from build123d import *

# Parameters (mm, degrees)
SKETCH_1_W                      = 90
SKETCH_1_H                      = 90
EXTRUDE_1_DEPTH                 = 15
SKETCH_2_W                      = 5
SKETCH_2_H                      = 82.5
CUT_EXTRUDE_1_DEPTH             = 102.734949747
CUT_EXTRUDE_2_REACH             = 67.383
SKETCH_3_W                      = 40
SKETCH_3_H                      = 90
FILLET_1_R                      = 10
CUT_EXTRUDE_3_DEPTH             = 65.420493634
EXTRUDE_4_DEPTH                 = 15
EXTRUDE_4_DEPTH_BACK            = 15
SKETCH_7_R                      = 5
EXTRUDE_5_DEPTH                 = 45
EXTRUDE_5_DEPTH_BACK            = 45
CUT_EXTRUDE_4_REACH             = 67.383
CUT_EXTRUDE_4_DIRECTION_2_DEPTH = 15
FILLET_2_R                      = 0.5
FILLET_3_R                      = 2


with BuildPart() as part:
    # 草图1 → 凸台-拉伸1 (new body)
    with BuildSketch(Plane(origin=(0, 0, 0), x_dir=(0, 0, -1), z_dir=(1, 0, 0))):
        Rectangle(SKETCH_1_W, SKETCH_1_H)
    extrude(amount=EXTRUDE_1_DEPTH)

    # 草图2 → 切除-拉伸1 (cut, through all)
    with BuildSketch(Plane.XY.offset(45)):
        with BuildLine():
            Line((0, 45), (0, 37.5))
            ThreePointArc((0, 37.5), (2.196699141, 42.803300859), (7.5, 45))
            Line((7.5, 45), (0, 45))
        make_face()
        with BuildLine():
            Line((15, 45), (7.5, 45))
            ThreePointArc((7.5, 45), (12.803300859, 42.803300859), (15, 37.5))
            Line((15, 37.5), (15, 45))
        make_face()
        with BuildLine():
            ThreePointArc((10, 37.5), (7.5, 40), (5, 37.5))
            Line((5, 37.5), (10, 37.5))
        make_face()
        with Locations((7.5, -3.75)):
            Rectangle(SKETCH_2_W, SKETCH_2_H)
    extrude(amount=-CUT_EXTRUDE_1_DEPTH, mode=Mode.SUBTRACT)

    # 切除-拉伸2: up to this face of the body (flat: up to its plane)
    cut_extrude_2_end = Plane(part.part.faces().sort_by_distance((5, -3.75, 0))[0])
    # 草图3 → 切除-拉伸2 (cut, up to the picked face)
    with BuildSketch(Plane(origin=(15, 0, 0), x_dir=(0, 0, -1), z_dir=(1, 0, 0)), mode=Mode.PRIVATE) as cut_extrude_2_sk1:
        Rectangle(SKETCH_3_W, SKETCH_3_H)
    cut_extrude_2_tool1 = split(extrude(cut_extrude_2_sk1.sketch, amount=-CUT_EXTRUDE_2_REACH, mode=Mode.PRIVATE), bisect_by=cut_extrude_2_end, keep=Keep.BOTH, mode=Mode.PRIVATE)
    add(cut_extrude_2_tool1.solids().sort_by(Axis((15, 0, 0), (-1, 0, 0)))[0], mode=Mode.SUBTRACT)

    # 圆角1
    fillet_1_edges = [part.edges().sort_by_distance(p)[0] for p in [
        (12.5, -45, 20),
        (12.5, -45, -20),
        (12.5, -45, -45),
        (12.5, -45, 45),
    ]]
    fillet(fillet_1_edges, radius=FILLET_1_R)

    # 草图4 → 切除-拉伸3 (cut, through all)
    with BuildSketch(Plane(origin=(5, 0, 0), x_dir=(0, 0, -1), z_dir=(1, 0, 0))):
        with BuildLine():
            Line((-20, 44.571067812), (-20, 37.104465858))
            ThreePointArc((-20, 37.104465858), (0, 17.104465858), (20, 37.104465858))
            Line((20, 37.104465858), (20, 44.571067812))
            Line((20, 44.571067812), (-20, 44.571067812))
        make_face()
    extrude(amount=-CUT_EXTRUDE_3_DEPTH, mode=Mode.SUBTRACT)

    # 草图7 → 凸台-拉伸4 (add, two sides: drawn at the far end of the back side and taken through both)
    with BuildSketch(Plane.XY.offset(-EXTRUDE_4_DEPTH_BACK)):
        with BuildLine():
            Line((0, -30), (-6, -30))
            ThreePointArc((-6, -30), (-13.5, -37.5), (-6, -45))
            Line((-6, -45), (0, -45))
            Line((0, -45), (0, -30))
        make_face()
        with Locations((-6, -37.5)):
            Circle(SKETCH_7_R, mode=Mode.SUBTRACT)
    extrude(amount=EXTRUDE_4_DEPTH + EXTRUDE_4_DEPTH_BACK)

    # 草图9 → 凸台-拉伸5 (add, two sides: drawn at the far end of the back side and taken through both)
    with BuildSketch(Plane.XY.offset(-EXTRUDE_5_DEPTH_BACK)):
        with BuildLine():
            Line((0, -24), (0, -30))
            Line((0, -30), (-6, -30))
            ThreePointArc((-6, -30), (-1.757359313, -28.242640687), (0, -24))
        make_face()
    extrude(amount=EXTRUDE_5_DEPTH + EXTRUDE_5_DEPTH_BACK)

    # 切除-拉伸4: up to this face of the body (flat: up to its plane)
    cut_extrude_4_end = Plane(part.part.faces().sort_by_distance((10, -2.920820113, 32.5))[0])
    # 草图6 → 切除-拉伸4 (cut, up to the picked face)
    with BuildSketch(Plane.ZY, mode=Mode.PRIVATE) as cut_extrude_4_sk1:
        with BuildLine():
            Line((45, 33.969795549), (45, -33.969795549))
            ThreePointArc((45, -33.969795549), (32.5, 0), (45, 33.969795549))
        make_face()
    cut_extrude_4_tool1 = split(extrude(cut_extrude_4_sk1.sketch, amount=-CUT_EXTRUDE_4_REACH, mode=Mode.PRIVATE), bisect_by=cut_extrude_4_end, keep=Keep.BOTH, mode=Mode.PRIVATE)
    # 草图6 → 切除-拉伸4 (cut, up to the picked face)
    with BuildSketch(Plane.ZY, mode=Mode.PRIVATE) as cut_extrude_4_sk2:
        with BuildLine():
            Line((-45, 33.969795549), (-45, -33.969795549))
            ThreePointArc((-45, -33.969795549), (-32.5, 0), (-45, 33.969795549))
        make_face()
    cut_extrude_4_tool2 = split(extrude(cut_extrude_4_sk2.sketch, amount=-CUT_EXTRUDE_4_REACH, mode=Mode.PRIVATE), bisect_by=cut_extrude_4_end, keep=Keep.BOTH, mode=Mode.PRIVATE)
    add(cut_extrude_4_tool1.solids().sort_by(Axis((0, 0, 39.945085), (1, 0, 0)))[0], mode=Mode.SUBTRACT)
    add(cut_extrude_4_tool2.solids().sort_by(Axis((0, 0, -39.945085), (1, 0, 0)))[0], mode=Mode.SUBTRACT)

    # 草图6 → 切除-拉伸4 direction 2 (cut)
    with BuildSketch(Plane.ZY):
        with BuildLine():
            Line((45, 33.969795549), (45, -33.969795549))
            ThreePointArc((45, -33.969795549), (32.5, 0), (45, 33.969795549))
        make_face()
        with BuildLine():
            Line((-45, 33.969795549), (-45, -33.969795549))
            ThreePointArc((-45, -33.969795549), (-32.5, 0), (-45, 33.969795549))
        make_face()
    extrude(amount=CUT_EXTRUDE_4_DIRECTION_2_DEPTH, mode=Mode.SUBTRACT)

    # 圆角2
    fillet_2_edges = [part.edges().sort_by_distance(p)[0] for p in [
        (-6, -30, -28.467980088),
        (-6, -30, 28.467980088),
    ]]
    fillet(fillet_2_edges, radius=FILLET_2_R)

    # 圆角3
    fillet_3_edges = [part.edges().sort_by_distance(p)[0] for p in [
        (0, -30, 28.467980088),
        (0, -30, -28.467980088),
    ]]
    fillet(fillet_3_edges, radius=FILLET_3_R)


solid = part.part
Build history of the part. All positions in model axes, mm. A direction names the side the tool comes from. Coordinates: 2 decimals unless noted, no trailing zeros. Order: outer loops, then holes, each group sorted by start corner. A loop starts at its lowest first (then second) coordinate and runs counter-clockwise, first axis right, second up. Notation, with made-up numbers: (15.5, -24.5) - (53.5, -24.5) arc R13 cw to (53.5, -7.5) - close; hole circle Ø11 at (65.5, 44). An arc over 180 degrees is marked (long way). Write each question's results on one line, items separated by ' | '. Start each with the question number.
Item 1: Flat gauge pins, fed straight in: pin 1 (3 mm diameter, centred on y = 14, z = 3, fed in from +X); pin 2 (18.5 mm diameter, centred on y = 14.5, z = -1.5, fed in from -X); pin 3 (12 mm diameter, centred on x = -3.5, y = -13, fed in from +Z). Where does each tip first touch, or does it go through?
Item 2: Tool access for faces 5 (the face through (12.54, -41.99, 42.15)), 6 (the face through (-0.57, -30.6, 29.4)), 7 (the face through (-8.3, -42.2, -15)), 8 (the face through (12.54, -41.99, -42.15)): list every direction of +Z, -Z, +X, -X, +Y, -Y with a clear straight run to the whole face (end or side of a thin tool).
Item 3: Wall check: probe 1 along Y at (x, z) = (-6, -7.75); probe 2 along Z at (x, y) = (13, 24.5); probe 3 along X at (y, z) = (-37, -3). Give the ranges that are in metal, low to high. Write a range as [from, to].
Item 4: Mould opens along X. For faces 1 (the face through (10, -4, -32)), 2 (the face through (10, -4, 33)), 3 (the face through (-1.123, -27.495, -0.578)), 4 (the face through (11, 13, -20)) say: released by +X, released by -X, zero draft, split by the parting line, or undercut.
Item 5: Band-saw the part on C-C on y = -37.5. Write the cut outline in (x, z).
Item 6: Band-saw the part on B-B on y = -21. Write the cut outline in (x, z).
Item 7: Band-saw the part on D-D on x = 2. Write the cut outline in (y, z), and give its area (3 significant figures).
Item 8: Band-saw the part on A-A on z = 0. Write the cut outline in (x, y).
Numbers:
1) pin 1: x = 5 | pin 2: x = 0 | pin 3: z = 35.64
2) face 5: +Z, +X, -Y | face 6: +Z, -X, -Y | face 7: -Z, -X, -Y | face 8: -Z, +X, -Y
3) probe 1: [-45, -42.5], [-32.5, -30] | probe 2: [-45, -20], [20, 45] | probe 3: [-13.48, -10.97], [-1.03, 5]
4) face 1: undercut | face 2: undercut | face 3: released by -X | face 4: zero draft
5) outline: (-13.5, -15) - (-11, -15) - (-11, 15) - (-13.5, 15) - close; (-1, -15) - (0, -15) - (0, -45) - (5, -45) - (5, 45) - (0, 45) - (0, 15) - (-1, 15) - close; (10, -44.68) - (15, -44.68) - (15, -20.32) - (10, -20.32) - close; (10, 20.32) - (15, 20.32) - (15, 44.68) - (10, 44.68) - close
6) outline: (0, -36.89) - (5, -36.89) - (5, 36.89) - (0, 36.89) - close; (10, -45) - (15, -45) - (15, -20) - (10, -20) - close; (10, 20) - (15, 20) - (15, 45) - (10, 45) - close
7) outline: (-45, -45) - (-33.97, -45) arc R52.41 cw to (33.97, -45) - (42.6, -45) - (42.6, -20) - (37.1, -20) arc R20 cw to (37.1, 20) - (42.6, 20) - (42.6, 45) - (33.97, 45) arc R52.41 cw to (-33.97, 45) - (-45, 45) - close | area: 5,870 mm^2
8) outline: (-6, -45) - (5, -45) - (5, 17.1) - (0, 17.1) - (0, -24) arc R6 cw to (-6, -30) arc R7.5 ccw to start; hole circle Ø10 at (-6, -37.5)
